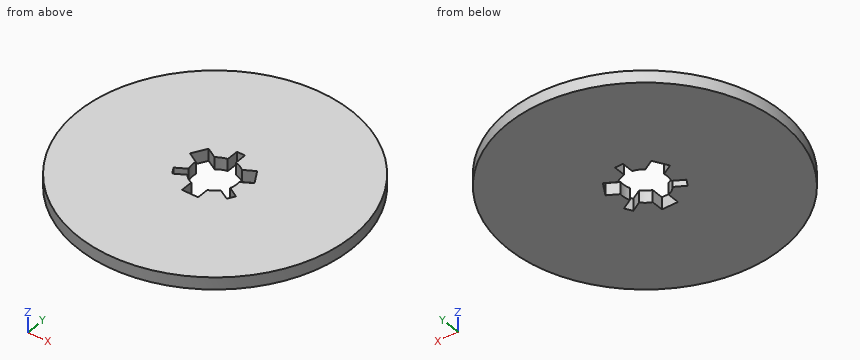
from build123d import *

# Parameters (mm, degrees)
SKETCH_R  = 34
PAD_DEPTH = 3


with BuildPart() as part:
    # Sketch → Pad (new body)
    with BuildSketch(Plane.XY):
        Circle(SKETCH_R)
        with BuildLine():
            ThreePointArc((3.43706, 4.293788), (2.287449, 5.001757), (1, 5.408327))
            Line((1, 8.408327), (1, 5.408327))
            Line((-1, 8.408327), (1, 8.408327))
            Line((-1, 5.408327), (-1, 8.408327))
            ThreePointArc((-1, 5.408327), (-2.287449, 5.001757), (-3.43706, 4.293788))
            Line((-6.035136, 5.793788), (-3.43706, 4.293788))
            Line((-8.035136, 2.329687), (-6.035136, 5.793788))
            Line((-5.43706, 0.829687), (-8.035136, 2.329687))
            ThreePointArc((-5.43706, 0.829687), (-5.475373, -0.51989), (-5.183748, -1.838138))
            Line((-7.781825, -3.338138), (-5.183748, -1.838138))
            Line((-6.781825, -5.070189), (-7.781825, -3.338138))
            Line((-4.183748, -3.570189), (-6.781825, -5.070189))
            ThreePointArc((-4.183748, -3.570189), (-3.187924, -4.481868), (-2, -5.123475))
            Line((-2, -8.123475), (-2, -5.123475))
            Line((2, -8.123475), (-2, -8.123475))
            Line((2, -5.123475), (2, -8.123475))
            ThreePointArc((2, -5.123475), (3.187924, -4.481868), (4.183748, -3.570189))
            Line((6.781825, -5.070189), (4.183748, -3.570189))
            Line((7.781825, -3.338138), (6.781825, -5.070189))
            Line((5.183748, -1.838138), (7.781825, -3.338138))
            ThreePointArc((5.183748, -1.838138), (5.475373, -0.51989), (5.43706, 0.829687))
            Line((8.035136, 2.329687), (5.43706, 0.829687))
            Line((6.035136, 5.793788), (8.035136, 2.329687))
            Line((3.43706, 4.293788), (6.035136, 5.793788))
        make_face(mode=Mode.SUBTRACT)
    extrude(amount=PAD_DEPTH)


solid = part.part
The model under review builds one solid part; all positions refer to its coordinate system, in mm. Coordinates: 2 decimals unless noted, no trailing zeros. Write each loop counter-clockwise with the first axis right and the second up, starting at its lowest first coordinate (ties: lowest second). Pieces come first, ordered by that corner, then holes. Notation, with made-up numbers: (8, 18) -> (14, 18) arc R15 cw to (14, 45) -> close; hole circle Ø2 at (-9, 68). An arc over 180 degrees is marked (long way). Answer in a Markdown table with one row per item.
1. Wall thickness on probe 1 along Y at (x, z) = (0, 2.4); probe 2 along X at (y, z) = (-4, 2.2); probe 3 along X at (y, z) = (-6, 2.75): over which ranges is each line inside the solid? List them lowest first. Write a range as [from, to].
Answers below:
| item | result |
|---|---|
| probe 1 | y = [-34, -8.12], [8.41, 34] |
| probe 2 | x = [-33.76, -7.4], [-4.93, -3.77], [3.77, 4.93], [7.4, 33.76] |
| probe 3 | x = [-33.47, -2], [2, 33.47] |
2. We need section A-A, the plane x = 0. State the section outline as (y, z) points.
Answers below:
| item | result |
|---|---|
| outline | (-34, 0) -> (-8.12, 0) -> (-8.12, 3) -> (-34, 3) -> close; (8.41, 0) -> (34, 0) -> (34, 3) -> (8.41, 3) -> close |
3. Clearance check with flat-ended pins moving along their axes: pin 1 Ø1 at (x, z) = (0.5, 2) entering from -Y; pin 2 Ø1.5 at (x, z) = (17.5, 1.5) entering from -Y; pin 3 Ø1.5 at (y, z) = (-6, 1) entering from -X. State where each tip first meets the part, or that it passes through.
Answers below:
| item | result |
|---|---|
| pin 1 | stops at y = -34 |
| pin 2 | stops at y = -29.59 |
| pin 3 | stops at x = -33.59 |
4. We need section C-C, the plane z = 1. State the section outline as (x, y) points.
Answers below:
| item | result |
|---|---|
| outline | circle Ø68 at (0, 0); hole (-8.04, 2.33) -> (-5.44, 0.83) arc R5.5 ccw to (-5.18, -1.84) -> (-7.78, -3.34) -> (-6.78, -5.07) -> (-4.18, -3.57) arc R5.5 ccw to (-2, -5.12) -> (-2, -8.12) -> (2, -8.12) -> (2, -5.12) arc R5.5 ccw to (4.18, -3.57) -> (6.78, -5.07) -> (7.78, -3.34) -> (5.18, -1.84) arc R5.5 ccw to (5.44, 0.83) -> (8.04, 2.33) -> (6.04, 5.79) -> (3.44, 4.29) arc R5.5 ccw to (1, 5.41) -> (1, 8.41) -> (-1, 8.41) -> (-1, 5.41) arc R5.5 ccw to (-3.44, 4.29) -> (-6.04, 5.79) -> close |
5. We need section B-B, the plane y = 0. State the section outline as (x, z) points, and give its area (3 significant figures).
Answers below:
| item | result |
|---|---|
| outline | (-34, 0) -> (-5.5, 0) -> (-5.5, 3) -> (-34, 3) -> close; (5.5, 0) -> (34, 0) -> (34, 3) -> (5.5, 3) -> close |
| area | 171 mm^2 |
6. We need section D-D, the plane x = 30. State the section outline as (y, z) points.
Answers below:
| item | result |
|---|---|
| outline | (-16, 0) -> (16, 0) -> (16, 3) -> (-16, 3) -> close |
